```python
from build123d import *

# Parameters (mm, degrees)
SKETCH1_W           = 112.72
SKETCH1_H           = 100
BOSS_EXTRUDE1_DEPTH = 6.36
SKETCH10_W          = 49.73
SKETCH10_H          = 6.36
CUT_EXTRUDE1_DEPTH  = 76.610179209
SKETCH11_W          = 6.36
SKETCH11_H          = 49.73
CUT_EXTRUDE2_DEPTH  = 76.610179209


with BuildPart() as part:
    # Sketch1 → Boss-Extrude1 (new body)
    with BuildSketch(Plane.XY):
        Rectangle(SKETCH1_W, SKETCH1_H)
    extrude(amount=BOSS_EXTRUDE1_DEPTH)

    # Sketch10 → Cut-Extrude1 (cut, through all)
    with BuildSketch(Plane.XY.offset(6.36)):
        with Locations((0, 46.82)):
            Rectangle(SKETCH10_W, SKETCH10_H)
    cut_extrude1 = extrude(amount=-CUT_EXTRUDE1_DEPTH, mode=Mode.SUBTRACT)

    # Mirror6: Cut-Extrude1 across plane
    add(cut_extrude1.mirror(Plane.ZX), mode=Mode.SUBTRACT)

    # Sketch11 → Cut-Extrude2 (cut, through all)
    with BuildSketch(Plane.XY.offset(6.36)):
        with Locations((53.18, 0)):
            Rectangle(SKETCH11_W, SKETCH11_H)
    cut_extrude2 = extrude(amount=-CUT_EXTRUDE2_DEPTH, mode=Mode.SUBTRACT)

    # Mirror7: Cut-Extrude2 across plane
    add(cut_extrude2.mirror(Plane(origin=(0, 0, 0), x_dir=(0, 0, 1), z_dir=(1, 0, 0))), mode=Mode.SUBTRACT)


solid = part.part
```
CAD build for the part. Positions are in the model's coordinates, mm. A direction names the side the tool comes from. Coordinates: 2 decimals unless noted, no trailing zeros. Order: outer loops, then holes, each group sorted by start corner. A loop starts at its lowest first (then second) coordinate and runs counter-clockwise, first axis right, second up. Notation, with made-up numbers: (34, 65.25) - (51, 65.25) arc R18 cw to (51, 92.25) - close; hole circle Ø5 at (50, 71). An arc over 180 degrees is marked (long way). Use a Markdown table: item, result. Add a question column.
(1) Pull direction X, two halves, no side cores. Call faces 4 (the face through (-24.865, 47, 3)), 5 (the face through (-50, 0, 3)), 6 (the face through (-41, 50, 3)): +X half, -X half, draft (parallel to the pull), parting line (faces both ways), or undercut.
(2) Saw through at C-C (y = -7.5). Give the cut face in (x, z), then the cut area to 3 significant figures.
(3) Saw through at B-B (x = 1.5). Give the cut face in (y, z).
(4) Which spindle directions (+Z, -Z, +X, -X, +Y, -Y) get a long thin tool onto all of the face, cutting with end or side? Do faces 1 (the face through (0, 43.64, 3)), 2 (the face through (-53, 24.865, 3)), 3 (the face through (-24.865, -47, 3)). Say none if no direction does.
(5) Flat gauge pins, fed straight in: pin 1 (1.9 mm diameter, centred on x = -5, z = 3, fed in from +Y); pin 2 (3 mm diameter, centred on y = -5, z = 2, fed in from -X); pin 3 (3 mm diameter, centred on y = -18.5, z = 4, fed in from +X). Where does each tip first touch, or does it go through?
(6) Saw through at A-A (z = 4.5). Give the cut face in (x, y) (3 decimals), then the cut area to 3 significant figures.
(7) Drill centre lines: line 1 along Y through (x, z) = (51, 5.75) (3 decimals); line 2 along Y through (x, z) = (-23, 3.25); line 3 along X through (y, z) = (4, 1.25). Where is each one in solid material? Low to high. Write a range as [from, to].
Solved:
| question | item | result |
|---|---|---|
| 1 | face 4 | undercut |
| 1 | face 5 | -X half |
| 1 | face 6 | draft |
| 2 | outline | (-50, 0) - (50, 0) - (50, 6.36) - (-50, 6.36) - close |
| 2 | area | 636 mm² |
| 3 | outline | (-43.64, 0) - (43.64, 0) - (43.64, 6.36) - (-43.64, 6.36) - close |
| 4 | face 1 | +Z, -Z, +Y |
| 4 | face 2 | +Z, -Z, -X |
| 4 | face 3 | +Z, -Z, -Y |
| 5 | pin 1 | stops at y = 43.64 |
| 5 | pin 2 | stops at x = -50 |
| 5 | pin 3 | stops at x = 50 |
| 6 | outline | (-56.36, -50) - (-24.865, -50) - (-24.865, -43.64) - (24.865, -43.64) - (24.865, -50) - (56.36, -50) - (56.36, -24.865) - (50, -24.865) - (50, 24.865) - (56.36, 24.865) - (56.36, 50) - (24.865, 50) - (24.865, 43.64) - (-24.865, 43.64) - (-24.865, 50) - (-56.36, 50) - (-56.36, 24.865) - (-50, 24.865) - (-50, -24.865) - (-56.36, -24.865) - close |
| 6 | area | 10,000 mm² |
| 7 | line 1 | y = [-50, -24.865], [24.865, 50] |
| 7 | line 2 | y = [-43.64, 43.64] |
| 7 | line 3 | x = [-50, 50] |
